Could you check a few things on this model? Use its own coordinates, in mm. A direction names the side the tool comes from. Give positions to 0.01 mm unless a question says otherwise; leave off trailing zeros. Write each loop counter-clockwise with the first axis right and the second up, starting at its lowest first coordinate (ties: lowest second). Pieces come first, ordered by that corner, then holes. Notation, with made-up numbers: M 0.5,30 L 40.5,30 A31 cw 40.5,62 Z; hole C 49,61.5 d8. An arc over 180 degrees is marked long. Use one line per item in the form item = value.
from build123d import *

# Parameters (mm, degrees)
SKETCH_W        = 84
SKETCH_H        = 71
PAD_DEPTH       = 130
SKETCH001_W     = 74
SKETCH001_H     = 71
POCKET_DEPTH    = 125
SKETCH002_R     = 8
PAD001_DEPTH    = 250
SKETCH003_R     = 2.1
SKETCH003_R_2   = 6.6
POCKET001_DEPTH = 84.001


with BuildPart() as part:
    # Sketch → Pad (new body)
    with BuildSketch(Plane.XY):
        Rectangle(SKETCH_W, SKETCH_H)
    extrude(amount=PAD_DEPTH)

    # Sketch001 → Pocket (cut)
    with BuildSketch(Plane.XY.offset(130)):
        Rectangle(SKETCH001_W, SKETCH001_H)
    extrude(amount=-POCKET_DEPTH, mode=Mode.SUBTRACT)

    # Sketch002 → Pad001 (new body)
    with BuildSketch(Plane(origin=(0, 0, 0), x_dir=(1, 0, 0), z_dir=(0, 0, -1))):
        Circle(SKETCH002_R)
    extrude(amount=PAD001_DEPTH)

    # Sketch003 → Pocket001 (cut, through all)
    with BuildSketch(Plane.YZ.offset(42)):
        with Locations((-20, 110)):
            Circle(SKETCH003_R)
        with Locations((20, 110)):
            Circle(SKETCH003_R)
        with Locations((0, 110)):
            Circle(SKETCH003_R_2)
        with Locations((0, 70)):
            Circle(SKETCH003_R)
        with Locations((-18.808843, 70)):
            Circle(SKETCH003_R)
        with Locations((18.808843, 70)):
            Circle(SKETCH003_R)
    extrude(amount=-POCKET001_DEPTH, mode=Mode.SUBTRACT)


solid = part.part
1) I want a section at C-C, the plane z = -104. Please give me the cut outline in (x, y).
Checked values:
outline = C 0,0 d16
2) I want a section at A-A, the plane x = 0. Please give me the cut outline in (y, z).
Checked values:
outline = M -35.5,0 L -8,0 L -8,-250 L 8,-250 L 8,0 L 35.5,0 L 35.5,5 L -35.5,5 Z
3) I want a section at D-D, the plane x = -16.5. Please give me the cut outline in (y, z), plus the area to 3 significant figures.
Checked values:
outline = M -35.5,0 L 35.5,0 L 35.5,5 L -35.5,5 Z
area = 355 mm2
4) I want a section at B-B, the plane y = -11.5. Please give me the cut outline in (x, z).
Checked values:
outline = M -42,0 L 42,0 L 42,130 L 37,130 L 37,5 L -37,5 L -37,130 L -42,130 Z
5) For faces 4 (the flat face through (-42, 0, 64)), 5 (the flat face through (37, -8, 68)), 6 (the cylindrical face through (-1.73, 7.81, -123.25)), which set-ups out of +Z, -Z, +X, -X, +Y, -Y let a thin tool reach every point of the face, with its end or its side?
Checked values:
face_4 = +Z, -Z, -X, +Y, -Y
face_5 = +Z, +Y, -Y
face_6 = -Z
6) Thinking about a two-plate mould opening in Y: for faces 1 (the cylindrical face through (39.535, -0.859, 116.544)), 2 (the flat face through (-38, -35.5, 55)), 3 (the flat face through (-0.6, 8.4, 0)), which applies, released by +Y, released by -Y, zero draft, split by the parting line, or undercut?
Checked values:
face_1 = undercut
face_2 = released by -Y
face_3 = zero draft
7) For pin 1 Ø1 at (y, z) = (-2.5, -79.5) entering from -X; pin 2 Ø4 at (x, z) = (1, -39.5) entering from +Y; pin 3 Ø4 at (x, y) = (27.5, -13) entering from +Z, each with a flat end and sliding along its axis, tell me the tip position at first contact or that it passes through.
Checked values:
pin_1 = -7.75
pin_2 = 8
pin_3 = 5
8) If I drill on L1, parallel to X at y = -11.5, z = 86; L2, parallel to Z at x = -40.3, y = -20; L3, parallel to Z at x = 10.5, y = -5, over which ranges is the centre line in solid material (lowest first)?
Checked values:
L1 = -42 to -37, 37 to 42
L2 = 0 to 68.27, 71.73 to 107.9, 112.1 to 130
L3 = 0 to 5
